Design review of the part built by this model. Coordinates are the model's own, in mm. A direction names the side the tool comes from. Round coordinates to 2 decimals unless told otherwise and drop trailing zeros. Write each question's results on one line, items separated by ' | '. Start each with the question number.
Item 1: Clearance check with flat-ended pins moving along their axes: pin 1 (2 mm diameter, centred on y = -53.5, z = 5, fed in from -X); pin 2 (14.5 mm diameter, centred on x = 0, y = -76.2, fed in from -Z); pin 3 (5 mm diameter, centred on x = 16, z = 7.5, fed in from -Y); pin 4 (4 mm diameter, centred on x = 6, z = 5.5, fed in from +Y). State where each tip first meets the part, or that it passes through.
Item 2: The part is to be moulded in two halves that separate along X. For faces 5 (the flat face through (0, -17, 12.7)), 6 (the cylindrical face through (14.864, -20.869, 6.261)), 7 (the cylindrical face through (-25.62, 0.24, 6.26)), 8 (the cylindrical face through (-23.087, -11.262, 6.261)), say which applies: +X half, -X half, draft (parallel to the pull), parting line (faces both ways), or undercut.
Item 3: Take a section at A-A, the plane z = 2.75. Count the separate pieces of the cut face and the enclosed holes in it, plus the area to 3 significant figures.
Item 4: Machinability: for faces 1 (the cylindrical face through (18.477, 17.845, 6.261)), 2 (the cylindrical face through (-11.262, 23.087, 6.261)), 3 (the cylindrical face through (20.869, 14.864, 6.261)), 4 (the cylindrical face through (-22.682, 12.058, 6.261)), which of the approach directions +Z, -Z, +X, -X, +Y, -Y give a long, thin tool a straight path to every point of the face, cutting with its end or side? Answer none if there is none.
Item 5: Wall thickness on line 1 (Y direction, x = -5, z = 1.5); line 2 (Y direction, x = -22, z = 9); line 3 (X direction, y = -34.5, z = 9.25): over which ranges is each line inside the solid? List them lowest first. Write a range as [from, to].
```python
from build123d import *

# Parameters (mm, degrees)
SKETCH3_R           = 27.94
GEARBODY_DEPTH      = 12.7
TOOTHCUT_DEPTH      = 13.7
CIRPATTERN1_COUNT   = 20
BOREDIA_R           = 6.35
BORE_DEPTH          = 12700
SKETCH4_R           = 6.35
BOSS_EXTRUDE1_DEPTH = 12.7


with BuildPart() as part:
    # Sketch3 → gearBody (new body)
    with BuildSketch(Plane.XY):
        Circle(SKETCH3_R)
    extrude(amount=GEARBODY_DEPTH)

    # Sketch2 → toothCut (cut, through all)
    with BuildSketch(Plane.XY):
        with BuildLine():
            ThreePointArc((22.161994813, -2.487872048), (22.207832173, -2.038556256), (22.244560977, -1.58840435))
            ThreePointArc((22.244560977, -1.58840435), (22.544698475, -0.941259068), (23.198766614, -0.656523398))
            ThreePointArc((23.198766614, -0.656523398), (27.638401864, 0.614170289), (31.045266607, 3.731588487))
            ThreePointArc((31.045266607, 3.731588487), (31.137815759, -2.858279396), (29.847095445, -9.321170787))
            ThreePointArc((29.847095445, -9.321170787), (27.064706273, -5.635613286), (22.930600611, -3.577897568))
            ThreePointArc((22.930600611, -3.577897568), (22.339300546, -3.17884398), (22.161994813, -2.487872048))
        make_face()
    toothcut = extrude(amount=TOOTHCUT_DEPTH, mode=Mode.SUBTRACT)

    # CirPattern1: toothCut ×20 about axis
    cirpattern1_axis = Axis((0, 0, 0), (0, 0, 1))
    for i in range(1, CIRPATTERN1_COUNT):
        add(toothcut.rotate(cirpattern1_axis, i * 360 / CIRPATTERN1_COUNT), mode=Mode.SUBTRACT)

    # boreDia → bore (cut, symmetric)
    with BuildSketch(Plane.XY):
        Circle(BOREDIA_R)
    extrude(amount=BORE_DEPTH, both=True, mode=Mode.SUBTRACT)

    # Sketch4 → Boss-Extrude1 (add)
    with BuildSketch(Plane.XY):
        with BuildLine():
            Line((-12.7, -18.331762639), (-12.7, -76.2))
            ThreePointArc((-12.7, -76.2), (0, -88.9), (12.7, -76.2))
            Line((12.7, -76.2), (12.7, -18.331762639))
            ThreePointArc((12.7, -18.331762639), (0, -22.3012), (-12.7, -18.331762639))
        make_face()
        with Locations((0, -76.2)):
            Circle(SKETCH4_R, mode=Mode.SUBTRACT)
    extrude(amount=BOSS_EXTRUDE1_DEPTH)


solid = part.part
```
Results list:
1) pin 1: x = -12.7 | pin 2: z = 0 | pin 3: y = -22.13 | pin 4: y = 27.32
2) face 5: draft | face 6: undercut | face 7: -X half | face 8: undercut
3) separate pieces: 1 | enclosed holes: 2 | area: 3,320 mm²
4) face 1: +Z, -Z, +Y | face 2: +Z, -Z | face 3: +Z, -Z, +X | face 4: +Z, -Z, -X
5) line 1: [-87.87, -80.11], [-72.29, -3.91], [3.91, 21.73] | line 2: [-17.22, -16.74], [-11.04, -6.39], [-4.12, 7.83], [11.42, 15.64] | line 3: [-12.7, 12.7]
